Source: three-view drawing plus pictorial views. Frame: mm from the lowest corner of the part. A direction names the side the tool comes from. Round coordinates to 2 decimals unless told otherwise and drop trailing zeros. Order: outer loops, then holes, each group sorted by start corner. A loop starts at its lowest first (then second) coordinate and runs counter-clockwise, first axis right, second up. Notation, with made-up numbers: M 32.5,4 L 58.5,4 A17 ccw 58.5,19 Z; hole C 45,-5.5 d8. An arc over 180 degrees is marked long. Return JSON: item names as keys, results as strings. Group by question number.
Q1. Ray query, probe 1 along Z at (x, y) = (11, 4.5); probe 2 along X at (y, z) = (2.75, 23); probe 3 along Y at (x, z) = (2, 29). Return the intervals inside material, ascending.
Q2. Cut plane B-B on z = 7. Output: boundary loops of the cut face in (x, y), and give its area (3 significant figures).
Q3. Cut plane D-D on y = 3.5. Output: boundary loops of the cut face in (x, z).
Q4. Cut plane A-A on y = 6. Output: boundary loops of the cut face in (x, z).
Q5. Cut plane C-C on x = 2.5. Output: boundary loops of the cut face in (y, z), and give its area (3 significant figures).
Q6. Contact query for flat-ended pins moving along their axis: pin 1 (2 mm diameter, centred on y = 8, z = 5, fed in from +X); pin 2 (4 mm diameter, centred on y = 3, z = 34.5, fed in from -X); pin 3 (5 mm diameter, centred on x = 5, z = 17.5, fed in from +Y); pin 4 (3 mm diameter, centred on x = 10, z = 24.5, fed in from -Y). Output: stop coordinate, or through.
Q7. Mould query, pull axis Z, two halves, no side actions, for the marked faces 1, 2 and 3. Classes: released by +Z, released by -Z, zero draft, split by the parting line, or undercut.
Q8. Access query for the marked faces 4, 5 and 6. Directions: +Z, -Z, +X, -X, +Y, -Y. A direction counts if a zero-diameter tool reaches every point of the face in a straight line with its end or side. Return the directions, or none.
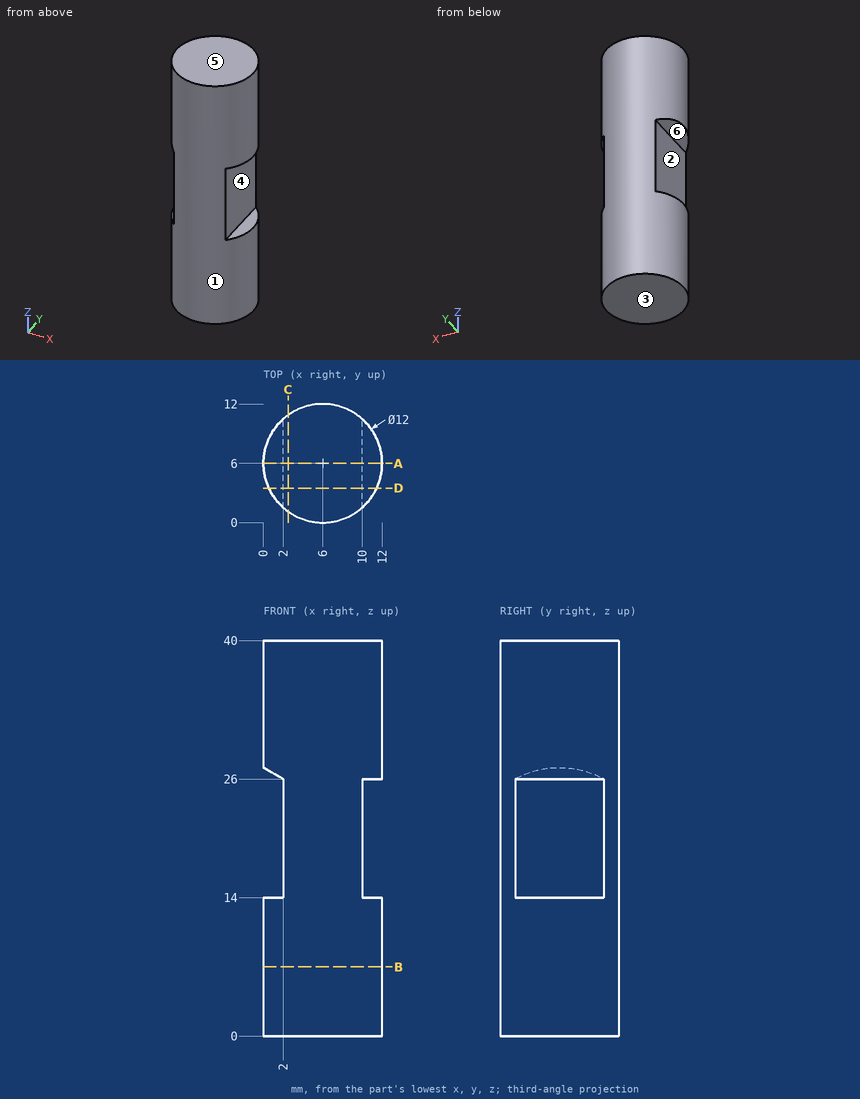
Result sheet:
{
 "1": {"probe 1": "z = 0 to 14, 26 to 40", "probe 2": "x = 2 to 10", "probe 3": "y = 1.53 to 10.47"},
 "2": {"outline": "C 6,6 d12", "area": "113 mm²"},
 "3": {"outline": "M 0.55,0 L 11.45,0 L 11.45,14 L 10,14 L 10,26 L 11.45,26 L 11.45,40 L 0.55,40 L 0.55,26.84 L 2,26 L 2,14 L 0.55,14 Z"},
 "4": {"outline": "M 0,0 L 12,0 L 12,14 L 10,14 L 10,26 L 12,26 L 12,40 L 0,40 L 0,27.15 L 2,26 L 2,14 L 0,14 Z"},
 "5": {"outline": "M 1.13,0 L 10.87,0 L 10.87,40 L 1.13,40 Z", "area": "390 mm²"},
 "6": {"pin 1": "stops at x = 11.92", "pin 2": "stops at x = 0.08", "pin 3": "stops at y = 12", "pin 4": "stops at y = 0.55"},
 "7": {"face 1": "zero draft", "face 2": "undercut", "face 3": "released by -Z"},
 "8": {"face 4": "+X, +Y, -Y", "face 5": "+Z, +X, -X, +Y, -Y", "face 6": "-X, +Y, -Y"}
}
